Part model, mm, in its own coordinate system. Face numbers are marked on the shaded views. A direction names the side the tool comes from. Give positions to 0.01 mm unless a question says otherwise; leave off trailing zeros. Order: outer loops, then holes, each group sorted by start corner. A loop starts at its lowest first (then second) coordinate and runs counter-clockwise, first axis right, second up. Notation, with made-up numbers: M -1.5,56 L 16.5,56 A12 cw 16.5,71 Z; hole C 42.25,15.25 d1. An arc over 180 degrees is marked long. Answer as a JSON object with one key per item and string values.
from build123d import *

# Parameters (mm, degrees)
SKETCH1_R           = 19.95
SKETCH1_R_2         = 13.05
BOSS_EXTRUDE1_DEPTH = 7
SKETCH2_R           = 13.05
SKETCH2_R_2         = 10
BOSS_EXTRUDE2_DEPTH = 1
SKETCH3_R           = 22
SKETCH3_R_2         = 13.05
BOSS_EXTRUDE3_DEPTH = 1
SKETCH4_R           = 22.5
SKETCH4_R_2         = 1.5
SKETCH4_R_3         = 13.05
BOSS_EXTRUDE7_DEPTH = 3
CHAMFER1_SIZE       = 1
SKETCH6_R           = 1.5
CUT_EXTRUDE1_DEPTH  = 1


with BuildPart() as part:
    # Sketch1 → Boss-Extrude1 (new body)
    with BuildSketch(Plane(origin=(0, 0, 0), x_dir=(1, 0, 0), z_dir=(0, 1, 0))):
        Circle(SKETCH1_R)
        Circle(SKETCH1_R_2, mode=Mode.SUBTRACT)
    extrude(amount=BOSS_EXTRUDE1_DEPTH)

    # Sketch2 → Boss-Extrude2 (add)
    with BuildSketch(Plane(origin=(0, 0, 0), x_dir=(-1, 0, 0), z_dir=(0, -1, 0))):
        Circle(SKETCH2_R)
        Circle(SKETCH2_R_2, mode=Mode.SUBTRACT)
    extrude(amount=-BOSS_EXTRUDE2_DEPTH)

    # Sketch3 → Boss-Extrude3 (add)
    with BuildSketch(Plane(origin=(0, 7, 0), x_dir=(1, 0, 0), z_dir=(0, 1, 0))):
        Circle(SKETCH3_R)
        Circle(SKETCH3_R_2, mode=Mode.SUBTRACT)
    extrude(amount=BOSS_EXTRUDE3_DEPTH)

    # Sketch4 → Boss-Extrude7 (add)
    with BuildSketch(Plane(origin=(0, 8, 0), x_dir=(1, 0, 0), z_dir=(0, 1, 0))):
        Circle(SKETCH4_R)
        with Locations((0, 19)):
            Circle(SKETCH4_R_2, mode=Mode.SUBTRACT)
        with Locations((19, 0)):
            Circle(SKETCH4_R_2, mode=Mode.SUBTRACT)
        with Locations((0, -19)):
            Circle(SKETCH4_R_2, mode=Mode.SUBTRACT)
        with Locations((-19, 0)):
            Circle(SKETCH4_R_2, mode=Mode.SUBTRACT)
        Circle(SKETCH4_R_3, mode=Mode.SUBTRACT)
    extrude(amount=BOSS_EXTRUDE7_DEPTH)

    # Chamfer1
    chamfer1_edges = [part.edges().sort_by_distance(p)[0] for p in [
        (-19.95, 0, 0),
        (-13.05, 11, 0),
    ]]
    chamfer(chamfer1_edges, length=CHAMFER1_SIZE)

    # Sketch6 → Cut-Extrude1 (cut)
    with BuildSketch(Plane(origin=(0, 8, 0), x_dir=(1, 0, 0), z_dir=(0, 1, 0))):
        with Locations((-19, 0)):
            Circle(SKETCH6_R)
        with Locations((0, -19)):
            Circle(SKETCH6_R)
        with Locations((19, 0)):
            Circle(SKETCH6_R)
        with Locations((0, 19)):
            Circle(SKETCH6_R)
    extrude(amount=-CUT_EXTRUDE1_DEPTH, mode=Mode.SUBTRACT)


solid = part.part
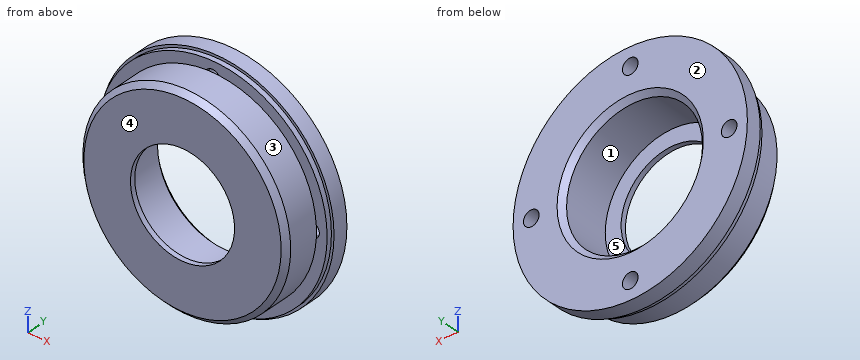
1. Two-plate mould, pull along X, no slides. Class the marked faces 3, 4 and 5: +X half, -X half, draft (parallel to the pull), parting line (faces both ways), or undercut.
Worked answers:
{"face 3": "parting line", "face 4": "draft", "face 5": "undercut"}
2. Pin check, flat tips, straight feed: P1, Ø4, axis at x = 2.5, y = 2, coming from the -Z side; P2, Ø1.5, axis at x = -2, y = 2, coming from the +Z side; P3, Ø1.2, axis at x = 0, z = 18.5, coming from the +Y side; P4, Ø15.5, axis at x = 0, z = 0, coming from the -Y side. Stop position of each tip, or through.
Worked answers:
{"P1": "stops at z = -19.94", "P2": "stops at z = 19.91", "P3": "stops at y = 7", "P4": "passes through"}
3. Cut at C-C on y = 5.5. Give the cut face in (x, z), plus the area to 3 significant figures.
Worked answers:
{"outline": "C 0,0 d39.9; hole C 0,0 d26.1", "area": "715 mm^2"}
4. Which spindle directions (+Z, -Z, +X, -X, +Y, -Y) get a long thin tool onto all of the face, cutting with end or side? Do the marked faces 1 and 2. Say none if no direction does.
Worked answers:
{"face 1": "+Y", "face 2": "+Z, -Z, +X, -X, +Y"}
5. Cut at A-A on x = 0. State how many separate pieces and enclosed holes the cut face has, plus the area to 3 significant figures.
Worked answers:
{"separate pieces": "4", "enclosed holes": "0", "area": "151 mm^2"}
6. Probe line 1 along X through (y, z) = (8.9, 0); line 2 along X through (y, z) = (7.45, 0). List the from-to ranges inside material, lowest first.
Worked answers:
{"line 1": "x = -22.5 to -20.5, -17.5 to -13.05, 13.05 to 17.5, 20.5 to 22.5", "line 2": "x = -22 to -20.5, -17.5 to -13.05, 13.05 to 17.5, 20.5 to 22"}
